```python
from build123d import *

# Parameters (mm, degrees)
F0_W      = 6
F0_H      = 6
F1_DEPTH  = 6
F1_FACE_W = 6
F1_FACE_H = 6
F5_W      = 6
F5_H      = 6
F6_DEPTH  = 6
F7_W      = 6
F7_H      = 6
F8_DEPTH  = 6


with BuildPart() as f1:
    # F0 (on Top) → F1 (new body)
    with BuildSketch(Plane.XY):
        with Locations((-3, 3)):
            Rectangle(F0_W, F0_H)
    extrude(amount=F1_DEPTH)

    # F3: sweep along a path in F2
    with BuildLine(Plane.XY) as f3_path:
        Line((0, 3.029319), (6, 3.029319))
    # F1_face (on face) → F3 (sweep)
    with BuildSketch(Plane(origin=(0, 3, 3), x_dir=(0, 1, 0), z_dir=(1, 0, 0))):
        Rectangle(F1_FACE_W, F1_FACE_H)
    sweep(path=f3_path.line)

    # F5 (on offset) → F6 (join)
    with BuildSketch(Plane.XY.offset(6)):
        with Locations((-3, 3)):
            Rectangle(F5_W, F5_H)
    extrude(amount=F6_DEPTH)

    # F7 (on Top) → F8 (join)
    with BuildSketch(Plane.XY):
        with Locations((-3, -3)):
            Rectangle(F7_W, F7_H)
    extrude(amount=F8_DEPTH)


solid = f1.part
```
Source: CAD feature listing. Evaluate the final solid. Frame: model axes, mm. A direction names the side the tool comes from. Coordinates: 2 decimals unless noted, no trailing zeros. Write each loop counter-clockwise with the first axis right and the second up, starting at its lowest first coordinate (ties: lowest second). Pieces come first, ordered by that corner, then holes. Notation, with made-up numbers: M 21.25,-30.75 L 63.25,-30.75 A23 cw 63.25,-18.75 Z; hole C -25.75,50.25 d4. An arc over 180 degrees is marked long. Answer as a JSON object with one key per item and string values.
1. Access query for faces 1 (the flat face through (0, 3, 9)), 2 (the flat face through (3, 0, 3)), 3 (the flat face through (-3, -6, 3)), 4 (the flat face through (-6, 1, 5)), 5 (the flat face through (-3, 0, 9)). Directions: +Z, -Z, +X, -X, +Y, -Y. A direction counts if a zero-diameter tool reaches every point of the face in a straight line with its end or side. Return the directions, or none.
Evaluation:
{"face 1": "+Z, +X, +Y, -Y", "face 2": "+Z, -Z, +X, -Y", "face 3": "+Z, -Z, +X, -X, -Y", "face 4": "+Z, -Z, -X, +Y, -Y", "face 5": "+Z, +X, -X, -Y"}
2. Contact query for flat-ended pins moving along their axis: P1, Ø5, axis at y = 4, z = 8, coming from the +X side; P2, Ø1.8, axis at x = -3, y = -4, coming from the +Z side; P3, Ø1.8, axis at x = 2.5, z = 2, coming from the -Y side; P4, Ø3, axis at y = 3, z = 10, coming from the +X side. Output: stop coordinate, or through.
Evaluation:
{"P1": "x = 6", "P2": "z = 6", "P3": "y = 0", "P4": "x = 0"}
3. Cut plane A-A on x = -4.25. Output: boundary loops of the cut face in (y, z), plus the area to 3 significant figures.
Evaluation:
{"outline": "M -6,0 L 6,0 L 6,12 L 0,12 L 0,6 L -6,6 Z", "area": "108 mm^2"}
4. Cut plane C-C on z = 11. Output: boundary loops of the cut face in (x, y).
Evaluation:
{"outline": "M -6,0 L 0,0 L 0,6 L -6,6 Z"}
5. Cut plane B-B on y = 4. Output: boundary loops of the cut face in (x, z).
Evaluation:
{"outline": "M -6,0 L 6,0 L 6,6 L 0,6 L 0,12 L -6,12 Z"}
6. Ray query, L1, parallel to Y at x = 0.5, z = 1.5; L2, parallel to X at y = -1.5, z = 1. Return the intervals inside material, ascending.
Evaluation:
{"L1": "0 to 6", "L2": "-6 to 0"}
